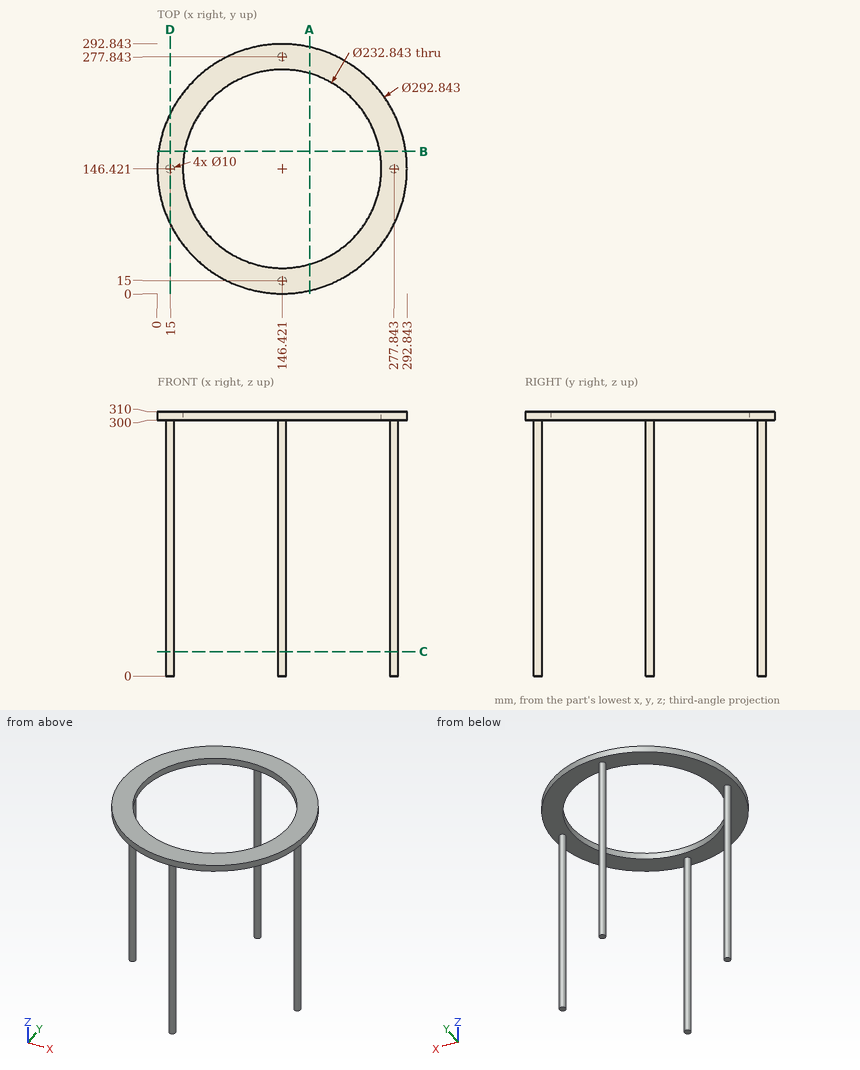
Can you work these out from the drawing? Everything is in mm from the part's minimum corner. Round coordinates to 2 decimals unless told otherwise and drop trailing zeros. Write each loop counter-clockwise with the first axis right and the second up, starting at its lowest first coordinate (ties: lowest second). Pieces come first, ordered by that corner, then holes.
1. I need wall thicknesses on L1, parallel to X at y = 277, z = 63; L2, parallel to Y at x = 148, z = 82 (1 decimal); L3, parallel to Z at x = 13, y = 158. Which ranges of each line are inside material? Lowest first, please.
2. Will this pin go through, and if not, where does the flat tip stop? pin 1 Ø6 at (x, y) = (66.5, 237.5) entering from -Z.
3. Suppose I cut it at A-A (x = 178.5). List the corners of the cut face in (y, z) for me (1 decimal).
4. Suppose I cut it at D-D (x = 15). List the corners of the cut face in (y, z) for me.
5. Suppose I cut it at B-B (y = 167). List the corners of the cut face in (x, z) for me.
6. Suppose I cut it at C-C (z = 28.5). List the corners of the cut face in (x, y) for me.
Answer sheet:
1. L1: x = 141.49 to 151.35
1. L2: y = 10.3 to 19.7, 273.1 to 282.6
1. L3: z = 300 to 310
2. pin 1: stops at z = 300
3. outline: (3.6, 300) - (34.5, 300) - (34.5, 310) - (3.6, 310) - close; (258.3, 300) - (289.3, 300) - (289.3, 310) - (258.3, 310) - close
4. outline: (81.86, 300) - (141.42, 300) - (141.42, 0) - (151.42, 0) - (151.42, 300) - (210.98, 300) - (210.98, 310) - (81.86, 310) - close
5. outline: (1.45, 300) - (31.83, 300) - (31.83, 310) - (1.45, 310) - close; (261.01, 300) - (291.39, 300) - (291.39, 310) - (261.01, 310) - close
6. outline: circle Ø10 at (15, 146.42); circle Ø10 at (146.42, 15); circle Ø10 at (146.42, 277.84); circle Ø10 at (277.84, 146.42)
